Autodesk Fusion 360 part; units mm, degrees
sketch "スケッチ16" plane through (0, 0, 0) normal (0, 0, 1) x (1, 0, 0)
  line L0 (8.0897, 44.9617) -> (8.1401, 76.9604)
  line L1 (0, 79.0322) -> (1.2, 79.0322)
  line L2 (0, 43.0322) -> (1.2, 43.0322)
  line L3 (0, 5) -> (0, 43.0322)
  arc A0 (5, 120) -> (0, 115) centre (5, 115) ccw
  line L4 (5, 120) -> (27.9289, 120)
  line L5 (137.9289, 0) -> (5, 0)
  arc A1 (0, 5) -> (5, 0) centre (5, 5) ccw
  line L6 (1.7, 75.5322) -> (1.2, 78.0322)
  line L7 (1.2, 43.0322) -> (1.2, 44.0322)
  line L8 (1.7, 75.5322) -> (4.7001, 75.5322)
  line L9 (1.2, 78.0322) -> (1.2, 79.0322)
  line L10 (10.1094, 86.7646) -> (10.1094, 107)
  line L11 (18.0897, 44.9502) -> (18.1401, 76.9623)
  line L12 (8.0897, 44.9617) -> (6.2705, 44.9617)
  arc A2 (18.1401, 76.9623) -> (10.1094, 86.7646) centre (8.1401, 76.9604) ccw
  line L13 (10, 35.1459) -> (10, 13)
  arc A3 (10, 35.1459) -> (18.0897, 44.9502) centre (8.0897, 44.9617) ccw
  arc A4 (49.7137, 74.7564) -> (62.3513, 73.5065) centre (56.7929, 81.8194) ccw
  line L14 (27.1123, 97.4097) -> (49.7137, 74.7564)
  arc A5 (24.1976, 104.8242) -> (27.1123, 97.4097) centre (34.1914, 104.4726) ccw
  line L15 (58.1413, 85.1894) -> (58.1413, 83.1647)
  line L16 (60.2627, 87.3108) -> (58.1413, 85.1894)
  line L17 (60.2627, 87.3108) -> (62.4073, 85.8948)
  line L18 (62.4073, 85.8948) -> (63.1023, 85.2006)
  line L19 (63.9508, 86.0492) -> (63.1023, 85.2006)
  line L20 (37.6352, 105.6955) -> (35.4143, 105.6955)
  line L21 (39.7566, 107.8168) -> (37.6352, 105.6955)
  line L22 (39.7566, 107.8168) -> (38.3423, 109.9382)
  line L23 (37.6465, 110.6565) -> (38.3423, 109.9382)
  line L24 (38.495, 111.505) -> (37.6465, 110.6565)
  line L25 (62.3513, 73.5065) -> (79.9289, 55.9289)
  line L26 (13.1094, 110) -> (19.2007, 110)
  line L27 (112.2124, 31.1183) -> (112.2124, 29.0936)
  line L28 (93.8389, 53.757) -> (91.7063, 51.6244)
  line L29 (88.2625, 50.4016) -> (110.864, 27.7483)
  line L30 (88.2625, 50.4016) -> (89.4854, 51.6244)
  line L31 (114.3337, 33.2397) -> (116.455, 31.8254)
  line L32 (114.3337, 33.2397) -> (112.2124, 31.1183)
  line L33 (91.7063, 51.6244) -> (89.4854, 51.6244)
  line L34 (91.7175, 56.5854) -> (92.4246, 55.8783)
  line L35 (81.1833, 43.3386) -> (103.7848, 20.6853)
  arc A6 (103.7848, 20.6853) -> (114.7117, 18.5182) centre (110.864, 27.7483) ccw
  line L36 (118.0236, 31.9764) -> (117.1751, 31.1279)
  arc A7 (79.9289, 55.9289) -> (81.1833, 43.3386) centre (88.2625, 50.4016) ccw
  line L37 (116.455, 31.8254) -> (117.1751, 31.1279)
  line L38 (93.8389, 53.757) -> (92.4246, 55.8783)
  line L39 (92.5661, 57.4339) -> (91.7175, 56.5854)
  line L40 (117.9874, 17.8705) -> (120.7365, 15.1213)
  arc A8 (13.1094, 110) -> (10.1094, 107) centre (13.1094, 107) ccw
  arc A9 (24.1976, 104.8242) -> (19.2007, 110) centre (19.2007, 105) ccw
  line L41 (118.6152, 10) -> (13, 10)
  arc A10 (10, 13) -> (13, 10) centre (13, 13) ccw
  arc A11 (118.6152, 10) -> (120.7365, 15.1213) centre (118.6152, 13) ccw
  line L42 (0, 79.0322) -> (0, 115)
  line L43 (38.495, 111.505) -> (31.4645, 118.5355)
  line L44 (63.9508, 86.0492) -> (92.5661, 57.4339)
  line L45 (118.0236, 31.9764) -> (141.4645, 8.5355)
  arc A12 (117.9874, 17.8705) -> (114.7117, 18.5182) centre (115.8661, 15.7491) ccw
  arc A13 (31.4645, 118.5355) -> (27.9289, 120) centre (27.9289, 115) ccw
  line L46 (4.7001, 75.5322) -> (6.1315, 76.9636)
  line L47 (4.7, 46.5322) -> (6.2705, 44.9617)
  arc A14 (137.9289, 0) -> (141.4645, 8.5355) centre (137.9289, 5) ccw
  line L48 (34.1914, 104.4726) -> (56.7929, 81.8194)
  line L49 (34.1914, 104.4726) -> (35.4143, 105.6955)
  line L50 (58.1413, 83.1647) -> (56.7929, 81.8194)
  line L51 (6.1315, 76.9636) -> (8.1401, 76.9604)
  line L52 (112.2124, 29.0936) -> (110.864, 27.7483)
  line L53 (4.7, 46.5322) -> (1.7, 46.5322)
  line L54 (1.7, 46.5322) -> (1.2, 44.0322)
  line L55 (8.0897, 44.9617) -> (8.1149, 60.9611)
extrude "押し出し1" add sketch "スケッチ16" along normal blind 20
hole "穴1" at (8.1149, 60.9611, 10) direction (1, -0.0016, 0) diameter 4.234 depth 13 tip angle 118
hole "穴2" at (99.5632, 39.0749, 10) direction (-0.7079, -0.7063, 0) diameter 4.234 depth 13 tip angle 118
hole "穴3" at (45.4922, 93.146, 10) direction (-0.7079, -0.7063, 0) diameter 4.234 depth 13 tip angle 118
hole "穴4" at (71.4645, 0, 10) direction (0, 1, 0) diameter 4.234 depth 13 tip angle 118
hole "穴5" at (33.0714, 0, 9.7195) direction (0, 1, 0) diameter 4.234 depth 13 tip angle 118
hole "穴6" at (16.4645, 120, 10) direction (0, -1, 0) diameter 3.332 depth 39 tip angle 180
Check sheet for the modelled part. Datum: model origin and axes. Units: mm. A direction names the side the tool comes from. Coordinates: 2 decimals unless noted, no trailing zeros. Write each loop counter-clockwise with the first axis right and the second up, starting at its lowest first coordinate (ties: lowest second). Pieces come first, ordered by that corner, then holes. Notation, with made-up numbers: (-31, 18) -> (18, 18) arc R15 ccw to (18, 44) -> close; hole circle Ø9 at (79, 48.5). An arc over 180 degrees is marked (long way). Use a Markdown table: item, result.
1. Sectioned sample at A-A (y = 70). Enter the section's corners in (x, z), plus the area to 3 significant figures.
Reported:
| item | result |
|---|---|
| outline | (8.13, 0) -> (18.13, 0) -> (18.13, 20) -> (8.13, 20) -> close; (65.86, 0) -> (80, 0) -> (80, 20) -> (65.86, 20) -> close |
| area | 483 mm2 |
2. Scan lines: line 1 along X through (y, z) = (33, 8.75); line 2 along X through (y, z) = (82.9, 10); line 3 along Y through (x, z) = (79, 3.25). Record each from-to range of solid material in increasing order.
Reported:
| item | result |
|---|---|
| line 1 | x = 0 to 10, 95.89 to 105.62, 114.09 to 114.69 |
| line 2 | x = 0 to 14.8, 41.59 to 55.71, 57.88 to 67.1 |
| line 3 | y = 0 to 10, 46.63 to 54.17, 56.86 to 71 |
3. Tool access check on faces 1 (the cylindrical face through (69.366, 5.07, 10.276)), 2 (the flat face through (3, 46.532, 10)), 3 (the cylindrical face through (55.9, 71.86, 9.86)), 4 (the flat face through (35, 115, 10)). Record the directions out of +Z, -Z, +X, -X, +Y, -Y that give a thin tool (end or side, any length) a straight path to the whole face; none if there is none.
Reported:
| item | result |
|---|---|
| face 1 | -Y |
| face 2 | +Z, -Z, -X |
| face 3 | +Z, -Z |
| face 4 | +Z, -Z, +X, +Y |
4. Go/stop test with flat-tipped pins: pin 1 Ø0.8 at (y, z) = (78.5, 6.5) entering from -X; pin 2 Ø7 at (x, z) = (33.07, 9.72) entering from +Y; pin 3 Ø1.3 at (x, z) = (1, 8) entering from -Y. Record where each tip stops, or that it passes through.
Reported:
| item | result |
|---|---|
| pin 1 | stops at x = 1.2 |
| pin 2 | stops at y = 119.72 |
| pin 3 | stops at y = 1.29 |
5. Release check for a two-part mould opening along Z. For faces 5 (the cylindrical face through (14.8, 82.3, 10)), 6 (the flat face through (3, 75.532, 10)) record: pulls with the +Z half, pulls with the -Z half, needs draft (parallel to the pull), parting line crosses it, or undercut.
Reported:
| item | result |
|---|---|
| face 5 | undercut |
| face 6 | needs draft |
